Read the model definition and answer for the solid it produces. Units are mm, in the model's axes. Give positions to 0.01 mm unless a question says otherwise; leave off trailing zeros. Order: outer loops, then holes, each group sorted by start corner. A loop starts at its lowest first (then second) coordinate and runs counter-clockwise, first axis right, second up.
Item 1: Find the intervals of material crossed by line 1 along Y through (x, z) = (106.5, 1.25); line 2 along X through (y, z) = (-1, 4.35); line 3 along X through (y, z) = (4, 1.2), in increasing order.
Item 2: The mould has two halves that part along Y. Classify faces 1 (the face through (149, 4, 3)), 2 (the face through (146.82, 0.11, 3.46)), 3 (the face through (-2, 0, 6)), 4 (the face through (108.807, -1.521, 2.958)): +Y half, -Y half, draft (parallel to the pull), parting line (faces both ways), or undercut.
Item 3: A cutting plane is placed at A-A (z = 4.65). Write down the section's boundary in (x, y), plus the area to 3 significant figures.
Item 4: Given pin 1 Ø4.5 at (x, y) = (106.82, 0) entering from -Z; pin 2 Ø1 at (y, z) = (-4.5, 3.5) entering from -X, each flat-ended and moving along its own axis, determine where each tip first touches the part or whether it passes through.
from build123d import *

# Parameters (mm, degrees)
SKETCH1_W           = 300
SKETCH1_H           = 12
BOSS_EXTRUDE1_DEPTH = 6
FILLET1_R           = 5
SKETCH2_R           = 2.5
CUT_EXTRUDE1_DEPTH  = 6
CHAMFER2_SIZE       = 1


with BuildPart() as part:
    # Sketch1 → Boss-Extrude1 (new body)
    with BuildSketch(Plane.XY):
        Rectangle(SKETCH1_W, SKETCH1_H)
    extrude(amount=BOSS_EXTRUDE1_DEPTH)

    # Fillet1
    fillet1_edges = [part.edges().sort_by_distance(p)[0] for p in [
        (150, -6, 3),
        (-150, -6, 3),
        (-150, 6, 3),
        (150, 6, 3),
    ]]
    fillet(fillet1_edges, radius=FILLET1_R)

    # Sketch2 → Cut-Extrude1 (cut)
    with BuildSketch(Plane(origin=(0, 0, 0), x_dir=(-1, 0, 0), z_dir=(0, 0, -1))):
        with Locations((-144.32263712, 0)):
            Circle(SKETCH2_R)
        with Locations((-106.82263712, 0)):
            Circle(SKETCH2_R)
    extrude(amount=-CUT_EXTRUDE1_DEPTH, mode=Mode.SUBTRACT)

    # Chamfer2
    chamfer2_edges = [part.edges().sort_by_distance(p)[0] for p in [
        (146.82263712, 0, 0),
    ]]
    chamfer(chamfer2_edges, length=CHAMFER2_SIZE)


solid = part.part
Response values:
1. line 1: y = -6 to -2.48, 2.48 to 6
1. line 2: x = -150 to 104.53, 109.11 to 142.03, 146.61 to 150
1. line 3: x = -149 to 149
2. face 1: +Y half
2. face 2: undercut
2. face 3: draft
2. face 4: undercut
3. outline: (-150, -1) arc R5 ccw to (-145, -6) - (145, -6) arc R5 ccw to (150, -1) - (150, 1) arc R5 ccw to (145, 6) - (-145, 6) arc R5 ccw to (-150, 1) - close; hole circle Ø5 at (106.82, 0); hole circle Ø5 at (144.32, 0)
3. area: 3,540 mm2
4. pin 1: passes through
4. pin 2: stops at x = -149
